```python
from build123d import *

# Parameters (mm, degrees)
SKETCH1_W           = 75
SKETCH1_H           = 75
SKETCH1_R           = 1.5
BOSS_EXTRUDE1_DEPTH = 6


with BuildPart() as part:
    # Sketch1 → Boss-Extrude1 (new body)
    with BuildSketch(Plane.XY):
        Rectangle(SKETCH1_W, SKETCH1_H)
        with Locations((-23.75, 23.75)):
            Circle(SKETCH1_R, mode=Mode.SUBTRACT)
        with Locations((23.75, 23.75)):
            Circle(SKETCH1_R, mode=Mode.SUBTRACT)
        with Locations((23.75, -23.75)):
            Circle(SKETCH1_R, mode=Mode.SUBTRACT)
        with Locations((-23.75, -23.75)):
            Circle(SKETCH1_R, mode=Mode.SUBTRACT)
        Polygon((-27.914213562, 13.772077939), (-13.772077939, 27.914213562), (13.772077939, 27.914213562), (27.914213562, 13.772077939), (27.914213562, -13.772077939), (13.772077939, -27.914213562), (-13.772077939, -27.914213562), (-27.914213562, -13.772077939), align=None, mode=Mode.SUBTRACT)
    extrude(amount=BOSS_EXTRUDE1_DEPTH)


solid = part.part
```
Design review of the part built by this model. Coordinates are the model's own, in mm. A direction names the side the tool comes from. Coordinates: 2 decimals unless noted, no trailing zeros. Order: outer loops, then holes, each group sorted by start corner. A loop starts at its lowest first (then second) coordinate and runs counter-clockwise, first axis right, second up.
1) Take a section at B-B, the plane z = 4.6. Give the boundary of the cut face in (x, y), and give its area (3 significant figures).
2) Take a section at C-C, the plane x = -18. Give the boundary of the cut face in (y, z).
3) Mouldability with a two-part tool opening along X and no side actions: class faces 3 (the flat face through (-17, 26, 0)), 4 (the flat face through (37.5, -1, 3)), 5 (the flat face through (-27.914, 0, 3)), 6 (the flat face through (-37.5, -1, 3)) as +X half, -X half, draft (parallel to the pull), parting line (faces both ways), or undercut.
4) Take a section at A-A, the plane y = 4. Give the boundary of the cut face in (x, z), and give its area (3 significant figures).
5) Wall thickness on line 1 along Y through (x, z) = (23.75, 3.55); line 2 along X through (y, z) = (-22.5, 4); line 3 along X through (y, z) = (-1.5, 0.2): over which ranges is each line inside the solid? List them lowest first.
6) Take a section at D-D, the plane x = 23.75. Give the boundary of the cut face in (y, z), and give its area (3 significant figures).
7) Clearance check with a flat-ended pin moving along its axis: pin 1 (2.5 mm diameter, centred on x = -23.75, y = -23.75, fed in from -Z). State where the tip first meets the part, or that it passes through.
8) For faces 1 (the flat face through (-17, 26, 6)), 2 (the flat face through (20.744, 20.942, 2.958)), list the 3-axis set-ups (+Z, -Z, +X, -X, +Y, -Y) from which the entire face can be reached by the end or side of a thin tool; tool diameter is ignored.
Returned:
1. outline: (-37.5, -37.5) - (37.5, -37.5) - (37.5, 37.5) - (-37.5, 37.5) - close; hole (-27.91, -13.77) - (-13.77, -27.91) - (13.77, -27.91) - (27.91, -13.77) - (27.91, 13.77) - (13.77, 27.91) - (-13.77, 27.91) - (-27.91, 13.77) - close; hole circle Ø3 at (-23.75, -23.75); hole circle Ø3 at (-23.75, 23.75); hole circle Ø3 at (23.75, -23.75); hole circle Ø3 at (23.75, 23.75)
1. area: 2,880 mm2
2. outline: (-37.5, 0) - (-23.69, 0) - (-23.69, 6) - (-37.5, 6) - close; (23.69, 0) - (37.5, 0) - (37.5, 6) - (23.69, 6) - close
3. face 3: draft
3. face 4: +X half
3. face 5: undercut
3. face 6: -X half
4. outline: (-37.5, 0) - (-27.91, 0) - (-27.91, 6) - (-37.5, 6) - close; (27.91, 0) - (37.5, 0) - (37.5, 6) - (27.91, 6) - close
4. area: 115 mm2
5. line 1: y = -37.5 to -25.25, -22.25 to -17.94, 17.94 to 22.25, 25.25 to 37.5
5. line 2: x = -37.5 to -24.58, -22.92 to -19.19, 19.19 to 22.92, 24.58 to 37.5
5. line 3: x = -37.5 to -27.91, 27.91 to 37.5
6. outline: (-37.5, 0) - (-25.25, 0) - (-25.25, 6) - (-37.5, 6) - close; (-22.25, 0) - (-17.94, 0) - (-17.94, 6) - (-22.25, 6) - close; (17.94, 0) - (22.25, 0) - (22.25, 6) - (17.94, 6) - close; (25.25, 0) - (37.5, 0) - (37.5, 6) - (25.25, 6) - close
6. area: 199 mm2
7. pin 1: passes through
8. face 1: +Z, +X, -X, +Y, -Y
8. face 2: +Z, -Z
